The listing builds one solid part. Answer for the finished solid, in the listing's coordinates (mm). A direction names the side the tool comes from. Give positions to 0.01 mm unless a question says otherwise; leave off trailing zeros. Loops run counter-clockwise (first coordinate to the right, second up) from the corner with the lowest first, then second, coordinate; pieces in that order, holes last. Notation, with made-up numbers: (8, -1.5) - (50, -1.5) arc R22 cw to (50, 30.5) - close; hole circle Ø1 at (82, 38.25). An arc over 180 degrees is marked (long way). Write each question's results on one line, items separated by ' | '.
Autodesk Inventor part; units mm, degrees
ref_plane "YZ Plane" through (0, 0, 0) normal (1, 0, 0) x (0, 1, 0)
ref_plane "XZ Plane" through (0, 0, 0) normal (0, 1, 0) x (-1, 0, 0)
ref_plane "XY Plane" through (0, 0, 0) normal (0, 0, 1) x (1, 0, 0)
sketch "Sketch1" plane through (0, 0, 0) normal (0, 1, 0) x (-1, 0, 0)
  line L0 (0, -11.2) -> (0, 11.2) construction
  line L1 (-11.2, 0) -> (11.2, 0) construction
  circle A0 centre (0, 0) radius 8
  dimension "d0" = 16
extrude "Extrusion1" add sketch "Sketch1" along normal blind 12
sketch "Sketch2" plane through (0, 12, 0) normal (0, 1, 0) x (1, 0, 0)
  circle A0 centre (0, 0) radius 6.5
  dimension "d3" = 13
extrude "Extrusion2" cut sketch "Sketch2" against normal blind 10
sketch "Sketch4" plane through (0, 0, 0) normal (0, -1, 0) x (1, 0, 0)
  line L0 (0, 11.2) -> (0, -11.2) construction
  line L1 (-11.2, 0) -> (11.2, 0) construction
  circle A0 centre (0, 5) radius 0.5
  circle A1 centre (0, -5) radius 0.5
  point P0 (0, 0)
  dimension "d39" = 1
  dimension "d40" = 1
  dimension "d41" = 10
extrude "Extrusion4" add sketch "Sketch4" along normal blind 9.5
equation "\"d40\" = d39"
properties part number "transducer"
Item 1: A cutting plane is placed at C-C, the plane y = -1.5. Determine the outline of the cut face in (x, z).
Values found:
outline: circle Ø1 at (0, -5); circle Ø1 at (0, 5)
Item 2: For faces 1 (the face through (0, 2, 0)), 2 (the face through (0, -9.5, 5)), 3 (the face through (-0.065, -4.684, -5.496)), determine the directions among +Z, -Z, +X, -X, +Y, -Y from which every point of the face is accessible in a straight line to the end or side of a thin tool.
Values found:
face 1: +Y | face 2: +Z, -Z, +X, -X, -Y | face 3: -Y
Item 3: A cutting plane is placed at B-B, the plane z = 0. Determine the outline of the cut face in (x, y), plus the area to 3 significant figures.
Values found:
outline: (-8, 0) - (8, 0) - (8, 12) - (6.5, 12) - (6.5, 2) - (-6.5, 2) - (-6.5, 12) - (-8, 12) - close | area: 62.0 mm²
Item 4: For a pull along X with two mould halves and no side action, classify faces 4 (the face through (0, 0, 0)), 5 (the face through (1.73, 5.92, 7.81)), 6 (the face through (-5.158, 7.07, 3.955)) as released by +X, released by -X, zero draft, split by the parting line, or undercut.
Values found:
face 4: zero draft | face 5: split by the parting line | face 6: undercut
Item 5: A cutting plane is placed at D-D, the plane y = 3. Determine the outline of the cut face in (x, z).
Values found:
outline: circle Ø16 at (0, 0); hole circle Ø13 at (0, 0)
Item 6: Flat-ended cylindrical pins translate along their axes: P1, Ø8, axis at x = 4, y = -0.5, coming from the +Z side; P2, Ø1.5, axis at x = -2.5, y = -3.5, coming from the -Z side; P3, Ø5, axis at y = -1.5, z = -3, coming from the +X side; P4, Ø1.5, axis at y = 5.5, z = 3.5, coming from the +X side. Find the tip coordinate at first contact, or state that the pin passes through.
Values found:
P1: stops at z = 8 | P2: passes through | P3: stops at x = 7.94 | P4: stops at x = 7.51
Item 7: Find the intervals of material crossed by line 1 along Z through (x, y) = (0, 4.5); line 2 along Z through (x, y) = (0, -5); line 3 along X through (y, z) = (6.75, 1.25), in increasing order. Write a range as [from, to].
Values found:
line 1: z = [-8, -6.5], [6.5, 8] | line 2: z = [-5.5, -4.5], [4.5, 5.5] | line 3: x = [-7.9, -6.38], [6.38, 7.9]
Item 8: A cutting plane is placed at A-A, the plane x = 0. Determine the outline of the cut face in (y, z), plus the area to 3 significant figures.
Values found:
outline: (-9.5, -5.5) - (0, -5.5) - (0, -8) - (12, -8) - (12, -6.5) - (2, -6.5) - (2, 6.5) - (12, 6.5) - (12, 8) - (0, 8) - (0, 5.5) - (-9.5, 5.5) - (-9.5, 4.5) - (0, 4.5) - (0, -4.5) - (-9.5, -4.5) - close | area: 81.0 mm²
